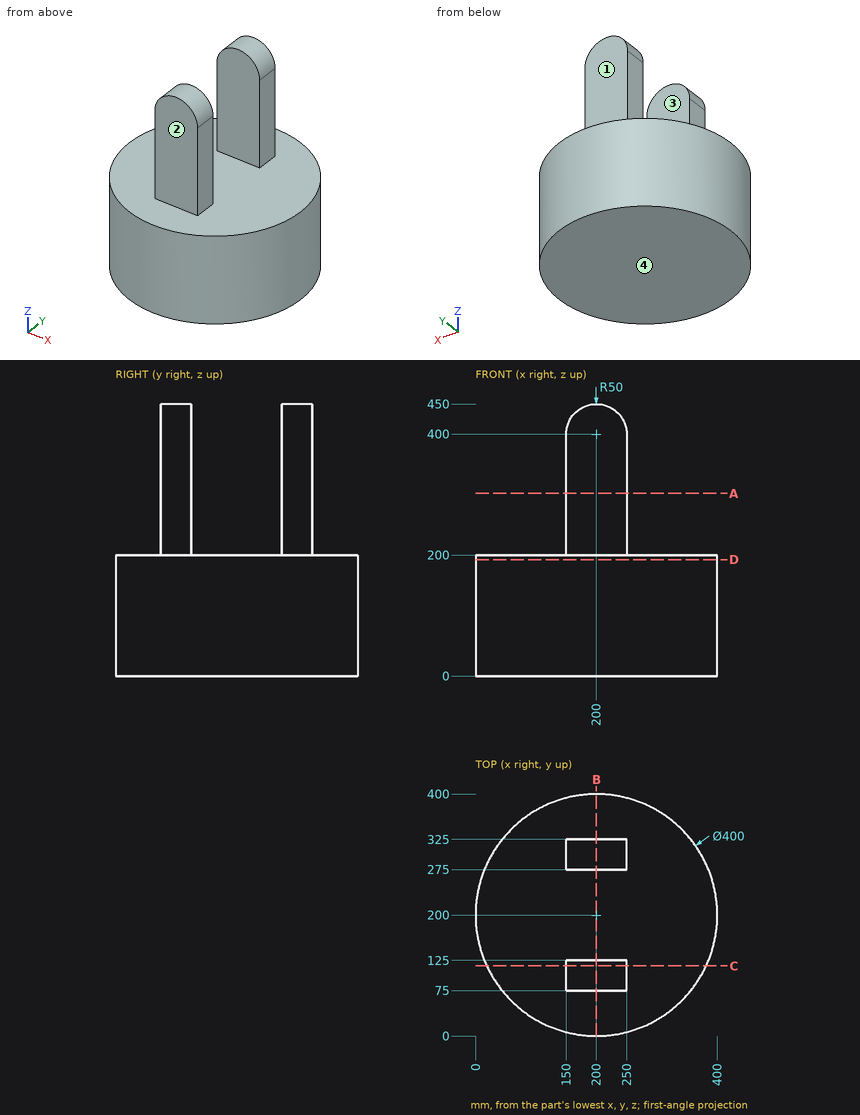
The figure shows three views and two pictorial views of one solid part (mm, origin at its lowest corner). Answer the questions. A direction names the side the tool comes from. Give positions to 0.01 mm unless a question says otherwise; leave off trailing zeros. Order: outer loops, then holes, each group sorted by start corner. A loop starts at its lowest first (then second) coordinate and runs counter-clockwise, first axis right, second up. Notation, with made-up numbers: (-22, 23) -> (-17, 23) arc R30 ccw to (-17, 55) -> close; hole circle Ø4 at (63.25, 10.25). An arc over 180 degrees is marked (long way). Write each question's results on one line, items separated by ' | '.
Q1. The part is cut by section B-B, the plane x = 200. Give the vertices of the cut face in (y, z).
Checked values:
outline: (0, 0) -> (400, 0) -> (400, 200) -> (325, 200) -> (325, 450) -> (275, 450) -> (275, 200) -> (125, 200) -> (125, 450) -> (75, 450) -> (75, 200) -> (0, 200) -> close
Q2. Straight lines are drawn through the part: probe 1 along Y at (x, z) = (246, 358.5); probe 2 along Z at (x, y) = (175, 381); probe 3 along X at (y, z) = (203, 19.5). For each, find the intervals that lie inside material, in ascending order. Write a range as from..to.
Checked values:
probe 1: y = 75..125, 275..325 | probe 2: z = 0..200 | probe 3: x = 0.02..399.98
Q3. Each of these flat-tipped pins is pushed along its axis until it touches: P1, Ø3, axis at x = 92.5, y = 51.5, coming from the -Z side; P2, Ø12, axis at y = 292, z = 66, coming from the -X side; P3, Ø5, axis at y = 302.5, z = 195, coming from the -X side; P4, Ø2, axis at x = 348, z = 127, coming from the -Y side. Where does it stop, or does it pass through?
Checked values:
P1: stops at z = 0 | P2: stops at x = 19.43 | P3: stops at x = 26.79 | P4: stops at y = 64.39
Q4. The part is cut by section A-A, the plane z = 302. Give the vertices of the cut face in (x, y).
Checked values:
outline: (150, 75) -> (250, 75) -> (250, 125) -> (150, 125) -> close; (150, 275) -> (250, 275) -> (250, 325) -> (150, 325) -> close
Q5. The part is cut by section C-C, the plane y = 116. Give the vertices of the cut face in (x, z).
Checked values:
outline: (18.5, 0) -> (381.5, 0) -> (381.5, 200) -> (250, 200) -> (250, 400) arc R50 ccw to (150, 400) -> (150, 200) -> (18.5, 200) -> close
Q6. The part is cut by section D-D, the plane z = 192.5. Give the vertices of the cut face in (x, y), and give its area (3 significant figures).
Checked values:
outline: circle Ø400 at (200, 200) | area: 126,000 mm^2
Q7. Which of the six approach directions +Z, -Z, +X, -X, +Y, -Y give full straight-line access (tool end or side, diameter ignored) to the marked faces 1, 2, 3 and 4?
Checked values:
face 1: +Z, +X, -X, +Y | face 2: +Z, +X, -X, -Y | face 3: +Z, +X, -X | face 4: -Z, +X, -X, +Y, -Y
